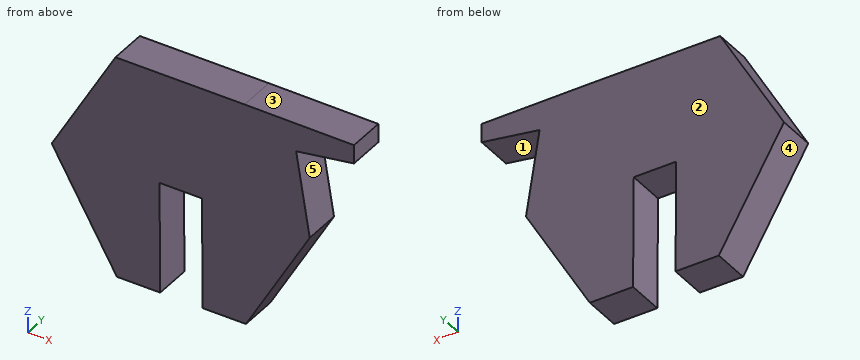
from build123d import *

# Parameters (mm, degrees)
BOSS_EXTRUDE1_DEPTH = 2.5
SKETCH2_W           = 2.85
SKETCH2_H           = 2.5
CUT_EXTRUDE1_DEPTH  = 7.5


with BuildPart() as part:
    # Sketch1 → Boss-Extrude1 (new body)
    with BuildSketch(Plane(origin=(0, 0, 0), x_dir=(1, 0, 0), z_dir=(0, 1, 0))):
        Polygon((12.694105225, -6.934131302), (12.694105225, -8.188855223), (5.34603962, -8.188855223), (-3.3140449, -8.134669239), (-7.59716072, -0.607723054), (-3.220192022, 6.865037146), (5.439892498, 6.810851162), (9.723008318, -0.716095023), (8.810324475, -6.299245302), align=None)
    extrude(amount=BOSS_EXTRUDE1_DEPTH)

    # Sketch2 → Cut-Extrude1 (cut)
    with BuildSketch(Plane(origin=(0.04282666, 0, -6.8446205), x_dir=(-0.999980426, 0, -0.006256859), z_dir=(0.006256859, 0, -0.999980426))):
        with Locations((-1.067171483, 1.25)):
            Rectangle(SKETCH2_W, SKETCH2_H)
    extrude(amount=-CUT_EXTRUDE1_DEPTH, mode=Mode.SUBTRACT)


solid = part.part
Model file for the job. Use its own axes, mm. Face numbers are marked on the shaded views. A direction names the side the tool comes from. Give positions to 0.01 mm unless a question says otherwise; leave off trailing zeros. Order: outer loops, then holes, each group sorted by start corner. A loop starts at its lowest first (then second) coordinate and runs counter-clockwise, first axis right, second up. Notation, with made-up numbers: M 7.5,-37 L 17.5,-37 A22 cw 17.5,0 Z; hole C 21,-21 d3. An arc over 180 degrees is marked long. Write item = value, one per line.
Q1. Cut at D-D, the plane x = 0. List the corners of the cut face in (y, z), then the cut area to 3 significant figures.
Derived:
outline = M 0,0.66 L 2.5,0.66 L 2.5,8.16 L 0,8.16 Z
area = 18.8 mm2
Q2. Tool access for the marked faces 1 and 2: list every direction of +Z, -Z, +X, -X, +Y, -Y with a clear straight run to the whole face (end or side of a thin tool).
Derived:
face_1 = +X, +Y, -Y
face_2 = +Z, -Z, +X, -X, +Y
Q3. Two-plate mould, pull along Z, no slides. Class the marked faces 3, 4 and 5: pulls with the +Z half, pulls with the -Z half, needs draft (parallel to the pull), parting line crosses it, or undercut.
Derived:
face_3 = pulls with the +Z half
face_4 = pulls with the -Z half
face_5 = undercut
Q4. Cut at B-B, the plane y = 0.4. List the corners of the cut face in (x, z) (3 decimals).
Derived:
outline = M -7.597,0.608 L -3.22,-6.865 L -0.315,-6.847 L -0.362,0.653 L 2.488,0.671 L 2.535,-6.829 L 5.44,-6.811 L 9.723,0.716 L 8.81,6.299 L 12.694,6.934 L 12.694,8.189 L 5.346,8.189 L -3.314,8.135 Z
Q5. Drill centre lines: line 1 (Z direction, x = 4.5, y = 0.2); line 2 (X direction, y = 1.5, z = -2.25); line 3 (X direction, y = 0.2, z = -2). Where is each one in solid material? Low to high. Write a range as [from, to].
Derived:
line_1 = [-6.82, 8.18]
line_2 = [-5.92, -0.34], [2.51, 8.04]
line_3 = [-6.07, -0.35], [2.5, 8.18]
Q6. Cut at C-C, the plane x = 9.5. List the corners of the cut face in (y, z), then the cut area to 3 significant figures.
Derived:
outline = M 0,0.32 L 2.5,0.32 L 2.5,2.08 L 0,2.08 Z; M 0,6.41 L 2.5,6.41 L 2.5,8.19 L 0,8.19 Z
area = 8.83 mm2
Q7. Flat gauge pin, fed straight in: pin 1 (1 mm diameter, centred on y = 2, z = 4, fed in from +X). Where does the tip first touch, or does it go through?
Derived:
pin_1 = 9.27
Q8. Cut at A-A, the plane z = -3.75. List the corners of the cut face in (x, y), then the cut area to 3 significant figures.
Derived:
outline = M -5.04,0 L -0.33,0 L -0.33,2.5 L -5.04,2.5 Z; M 2.52,0 L 7.18,0 L 7.18,2.5 L 2.52,2.5 Z
area = 23.4 mm2
